from build123d import *

# Parameters (mm, degrees)
SKETCH1_R               = 31.25
BOSS_EXTRUDE1_DEPTH     = 2
SKETCH2_W               = 38
SKETCH2_H               = 26
BOSS_EXTRUDE2_DEPTH     = 48
SKETCH3_W               = 34
SKETCH3_H               = 38
CUT_EXTRUDE1_DEPTH      = 48
CUT_EXTRUDE2_DEPTH      = 48
M12X1_25_TAPPED_HOLE1_D = 10.8
SKETCH7_W               = 2
SKETCH7_H               = 6
CUT_EXTRUDE3_DEPTH      = 48
FILLET2_R               = 1
SKETCH8_R               = 9
BOSS_EXTRUDE3_DEPTH     = 87.5


with BuildPart() as part:
    # Sketch1 → Boss-Extrude1 (new body)
    with BuildSketch(Plane(origin=(0, 0, 0), x_dir=(1, 0, 0), z_dir=(0, 1, 0))):
        with Locations(Location((0, 0, 0), (0, 0, 270))):
            Circle(SKETCH1_R)
    extrude(amount=BOSS_EXTRUDE1_DEPTH)

    # Sketch2 → Boss-Extrude2 (add)
    with BuildSketch(Plane.XZ):
        Rectangle(SKETCH2_W, SKETCH2_H)
    extrude(amount=BOSS_EXTRUDE2_DEPTH)

    # Sketch3 → Cut-Extrude1 (cut)
    with BuildSketch(Plane.XY.offset(13)):
        with Locations((0, -29)):
            Rectangle(SKETCH3_W, SKETCH3_H)
    extrude(amount=-CUT_EXTRUDE1_DEPTH, mode=Mode.SUBTRACT)

    # Sketch4 → Cut-Extrude2 (cut)
    with BuildSketch(Plane(origin=(19, 0, 0), x_dir=(0, 0, -1), z_dir=(1, 0, 0))):
        with BuildLine():
            ThreePointArc((0, -48), (-9.192388155, -44.192388155), (-13, -35))
            Line((-13, -35), (-13, -48))
            Line((-13, -48), (0, -48))
        make_face()
        with BuildLine():
            Line((13, -48), (13, -35))
            ThreePointArc((13, -35), (9.192388155, -44.192388155), (0, -48))
            Line((0, -48), (13, -48))
        make_face()
    extrude(amount=-CUT_EXTRUDE2_DEPTH, mode=Mode.SUBTRACT)

    # M12x1.25 Tapped Hole1 (through all)
    with Locations(Plane(origin=(19, 0, 0), x_dir=(0, 0, -1), z_dir=(1, 0, 0))):
        with Locations((0, -35)):
            Hole(M12X1_25_TAPPED_HOLE1_D / 2)

    # Sketch7 → Cut-Extrude3 (cut)
    with BuildSketch(Plane(origin=(0, 0, -13), x_dir=(-1, 0, 0), z_dir=(0, 0, -1))):
        with Locations((-18, -5)):
            Rectangle(SKETCH7_W, SKETCH7_H)
        with Locations((18, -5)):
            Rectangle(SKETCH7_W, SKETCH7_H)
    extrude(amount=-CUT_EXTRUDE3_DEPTH, mode=Mode.SUBTRACT)

    # Fillet2
    fillet2_edges = [part.edges().sort_by_distance(p)[0] for p in [
        (17, -10, 0),
        (-17, -10, 0),
        (19, -8, 0),
        (17, -8, 0),
        (17, -2, 0),
        (19, -2, 0),
        (19, 0, 0),
        (-19, 0, 0),
        (-19, -2, 0),
        (-17, -2, 0),
        (-17, -8, 0),
        (-19, -8, 0),
    ]]
    fillet(fillet2_edges, radius=FILLET2_R - 0.0001)  # a hair under: the kernel refuses the full size

    # Sketch8 → Boss-Extrude3 (add)
    with BuildSketch(Plane(origin=(0, 2, 0), x_dir=(1, 0, 0), z_dir=(0, 1, 0))):
        with Locations(Location((0, 0, 0), (0, 0, 270))):
            Circle(SKETCH8_R)
    extrude(amount=BOSS_EXTRUDE3_DEPTH)


solid = part.part
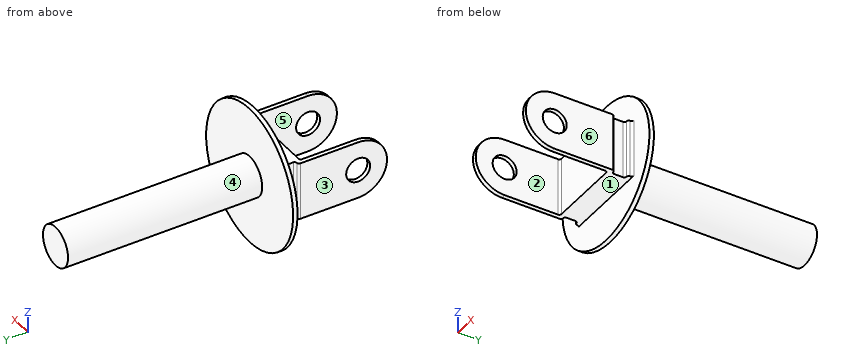
Check sheet for the modelled part. Datum: model origin and axes. Units: mm. Face numbers are marked on the shaded views. A direction names the side the tool comes from. Give positions to 0.01 mm unless a question says otherwise; leave off trailing zeros. Loops run counter-clockwise (first coordinate to the right, second up) from the corner with the lowest first, then second, coordinate; pieces in that order, holes last. Notation, with made-up numbers: M -11.75,11 L 19.25,11 A23 ccw 19.25,37 Z; hole C 48.5,43 d3. An arc over 180 degrees is marked long. Answer as a JSON object with one key per item and string values. Group by question number.
Q1. Material ranges on line 1 along Y through (x, z) = (-18.5, -3.5); line 2 along Y through (x, z) = (-9.5, -28); line 3 along X through (y, z) = (-5.5, -8), recorded low to high. Write a range as [from, to].
Q2. Access from +Z, -Z, +X, -X, +Y, -Y to the whole of each face (thin tool, end or side, straight path). Record for the marked faces 4, 5 and 6.
Q3. Cross-section at A-A on x = 0. Record the cut outline in (y, z).
Q4. Cross-section at C-C on z = -2. Give the number of separate pieces and of enclosed holes in the cut face, then the cut area to 3 significant figures.
Q5. Cross-section at D-D on z = 25. Record the cut outline in (x, y).
Q6. Cross-section at B-B on y = 79.5. Record the cut outline in (x, z), then the cut area to 3 significant figures.
Q7. Go/stop test with flat-tipped pins: P1, Ø10, axis at y = -23, z = -14.5, coming from the -X side; P2, Ø5, axis at x = -6.5, z = -11, coming from the -Y side; P3, Ø19, axis at x = 6.5, z = -10, coming from the +Y side; P4, Ø1.5, axis at x = -17, z = 6, coming from the +Y side. Record where each tip stops, or that it passes through.
Q8. Release check for a two-part mould opening along X. For the marked faces 1, 2 and 3 record: released by +X, released by -X, zero draft, split by the parting line, or undercut.
Evaluation:
{
 "1": {"line 1": "y = [-47.52, -39.11], [-30.89, -8.13], [-1.87, 2]", "line 2": "y = [0, 2]", "line 3": "x = [-17, 17]"},
 "2": {"face 4": "+Y", "face 5": "+Z, -Z, -Y", "face 6": "+Z, -Z, +X, -Y"},
 "3": {"outline": "M -10,-13 L 0,-13 L 0,-31.25 L 2,-31.25 L 2,-9 L 89.5,-9 L 89.5,9 L 2,9 L 2,31.25 L 0,31.25 L 0,13 L -10,13 Z"},
 "4": {"separate pieces": "3", "enclosed holes": "0", "area": "2,130 mm2"},
 "5": {"outline": "M -18.75,0 L 18.75,0 L 18.75,2 L -18.75,2 Z"},
 "6": {"outline": "C 0,0 d18", "area": "254 mm2"},
 "7": {"P1": "stops at x = -19", "P2": "stops at y = -10", "P3": "stops at y = 89.5", "P4": "stops at y = 2"},
 "8": {"face 1": "zero draft", "face 2": "undercut", "face 3": "released by -X"}
}
